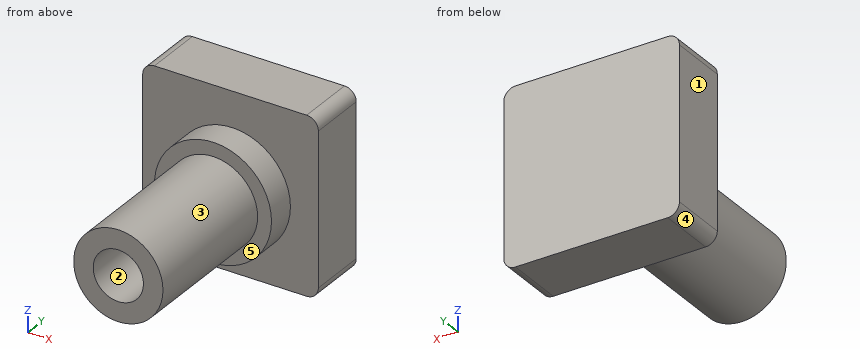
from build123d import *

# Parameters (mm, degrees)
F0_W     = 76.2
F0_H     = 76.2
F1_DEPTH = 25.4
F2_R     = 5.08
F3_R     = 25.383662
F4_DEPTH = 12.7
F5_R     = 19.36967
F6_DEPTH = 63.5
F7_R     = 10.899394
F8_DEPTH = 63.5


with BuildPart() as f1:
    # F0 (on Front) → F1 (new body)
    with BuildSketch(Plane.XZ):
        with Locations((4.244136, 2.642533)):
            Rectangle(F0_W, F0_H)
    extrude(amount=F1_DEPTH)

    # F2
    f2_edges = [f1.edges().sort_by_distance(p)[0] for p in [
        (-33.855864, -12.7, 40.742533),
        (42.344136, -12.7, 40.742533),
        (42.344136, -12.7, -35.457467),
        (-33.855864, -12.7, -35.457467),
    ]]
    fillet(f2_edges, radius=F2_R)

    # F3 (on face) → F4 (join)
    with BuildSketch(Plane.XZ.offset(25.4)):
        with Locations((4.844644, 0)):
            Circle(F3_R)
    extrude(amount=F4_DEPTH)

    # F5 (on face) → F6 (join)
    with BuildSketch(Plane.XZ.offset(38.1)):
        with Locations((4.844644, 0)):
            Circle(F5_R)
    extrude(amount=F6_DEPTH)

    # F7 (on face) → F8 (cut)
    with BuildSketch(Plane.XZ.offset(101.6)):
        with Locations((4.844644, 0)):
            Circle(F7_R)
    extrude(amount=-F8_DEPTH, mode=Mode.SUBTRACT)


solid = f1.part
Work out the finished part from the listing and answer in its coordinate system (mm). Face numbers are marked on the shaded views. A direction names the side the tool comes from. Give positions to 0.01 mm unless a question says otherwise; leave off trailing zeros. Loops run counter-clockwise (first coordinate to the right, second up) from the corner with the lowest first, then second, coordinate; pieces in that order, holes last. Notation, with made-up numbers: (70, 54.5) -> (122, 54.5) arc R15 cw to (122, 70.5) -> close; hole circle Ø1 at (64.25, 20). An arc over 180 degrees is marked (long way). Use a Markdown table: item, result. Add a question column.
1. Section C-C on x = 26 is taken. Determine the outline of the cut face in (y, z), and give its area (3 significant figures).
2. Determine the mould class of the marked faces 1, 2 and 3 for opening direction Z: released by +Z, released by -Z, zero draft, split by the parting line, or undercut.
3. Flat-ended cylindrical pins translate along their axes: pin 1 Ø8 at (y, z) = (-46.5, -7.5) entering from +X; pin 2 Ø6 at (y, z) = (-76, -19) entering from -X; pin 3 Ø6.5 at (x, z) = (1.5, -4) entering from -Y. Find the tip coordinate at first contact, or state that the pin passes through.
4. Section D-D on x = 3 is taken. Determine the outline of the cut face in (y, z), and give its area (3 significant figures).
5. Section A-A on z = 0 is taken. Determine the outline of the cut face in (x, y).
6. Section B-B on y = -56 is taken. Determine the outline of the cut face in (x, z).
7. For the marked faces 4 and 5, determine the directions among +Z, -Z, +X, -X, +Y, -Y from which every point of the face is accessible in a straight line to the end or side of a thin tool.
8. Find the intervals of material crossed by probe 1 along Y at (x, z) = (-13.5, 33.5); probe 2 along Y at (x, z) = (6, 10); probe 3 along Z at (x, y) = (1, -95), in increasing order.
Results below:
| question | item | result |
|---|---|---|
| 1 | outline | (-38.1, -14.03) -> (-25.4, -14.03) -> (-25.4, -35.46) -> (0, -35.46) -> (0, 40.74) -> (-25.4, 40.74) -> (-25.4, 14.03) -> (-38.1, 14.03) -> close |
| 1 | area | 2,290 mm^2 |
| 2 | face 1 | zero draft |
| 2 | face 2 | undercut |
| 2 | face 3 | split by the parting line |
| 3 | pin 1 | stops at x = 23.9 |
| 3 | pin 2 | stops at x = -6.07 |
| 3 | pin 3 | stops at y = -38.1 |
| 4 | outline | (-101.6, -19.28) -> (-38.1, -19.28) -> (-38.1, -25.32) -> (-25.4, -25.32) -> (-25.4, -35.46) -> (0, -35.46) -> (0, 40.74) -> (-25.4, 40.74) -> (-25.4, 25.32) -> (-38.1, 25.32) -> (-38.1, 19.28) -> (-101.6, 19.28) -> (-101.6, 10.74) -> (-38.1, 10.74) -> (-38.1, -10.74) -> (-101.6, -10.74) -> close |
| 4 | area | 3,660 mm^2 |
| 5 | outline | (-33.86, -25.4) -> (-20.54, -25.4) -> (-20.54, -38.1) -> (-14.53, -38.1) -> (-14.53, -101.6) -> (-6.05, -101.6) -> (-6.05, -38.1) -> (15.74, -38.1) -> (15.74, -101.6) -> (24.21, -101.6) -> (24.21, -38.1) -> (30.23, -38.1) -> (30.23, -25.4) -> (42.34, -25.4) -> (42.34, 0) -> (-33.86, 0) -> close |
| 6 | outline | circle Ø38.74 at (4.84, 0); hole circle Ø21.8 at (4.84, 0) |
| 7 | face 4 | -Z, -X, +Y, -Y |
| 7 | face 5 | -Y |
| 8 | probe 1 | y = -25.4 to 0 |
| 8 | probe 2 | y = -38.1 to 0 |
| 8 | probe 3 | z = -18.98 to -10.2, 10.2 to 18.98 |
